Check sheet for the drawn part. Datum: minimum x, y, z corner. Units: mm. A direction names the side the tool comes from. Give positions to 0.01 mm unless a question says otherwise; leave off trailing zeros. Order: outer loops, then holes, each group sorted by start corner. A loop starts at its lowest first (then second) coordinate and runs counter-clockwise, first axis right, second up.
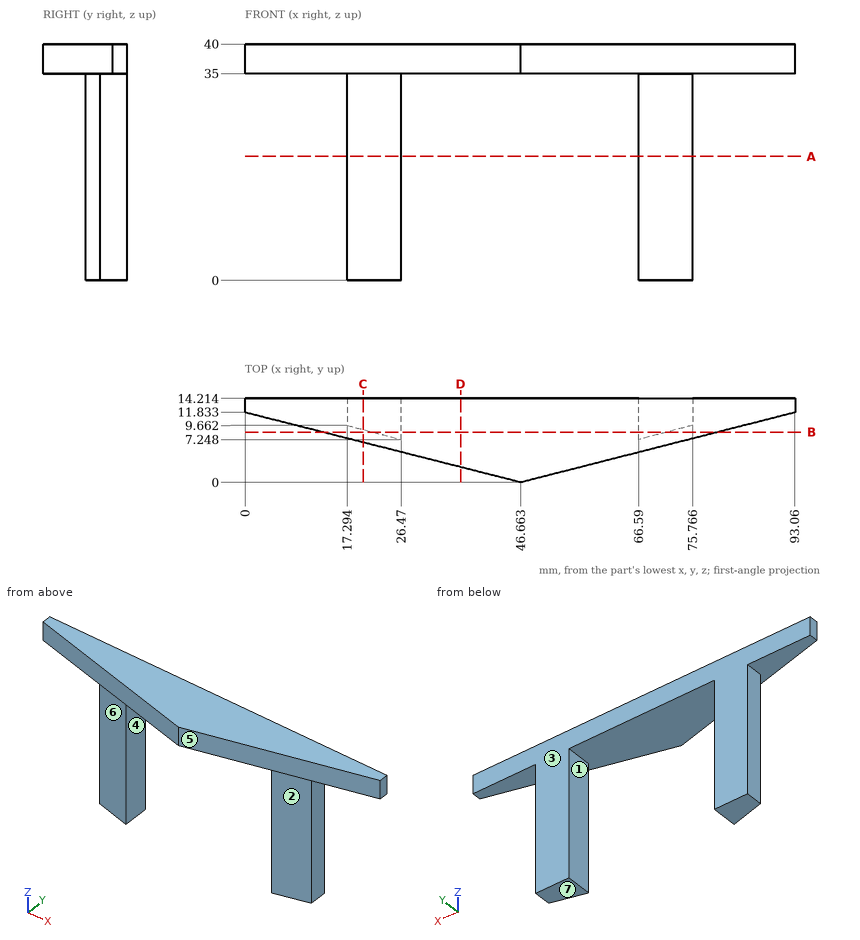
(1) Section check D-D, the plane x = 36.5. Enter the section's corners in (y, z), then the cut area to 3 significant figures.
Solved:
outline: (2.58, 35) - (14.21, 35) - (14.21, 40) - (2.58, 40) - close
area: 58.2 mm2
(2) Section check C-C, the plane x = 20. Enter the section's corners in (y, z).
Solved:
outline: (6.76, 35) - (8.95, 35) - (8.95, 0) - (14.21, 0) - (14.21, 40) - (6.76, 40) - close
(3) Set-up check for the marked faces 1, 2 and 3: record each of +Z, -Z, +X, -X, +Y, -Y from which the full face is reachable in a straight line by a thin tool's end or side.
Solved:
face 1: -Z, +Y, -Y
face 2: -Z, +X, -Y
face 3: +Z, -Z, +X, -X, +Y
(4) Section check A-A, the plane z = 21. Enter the section's corners in (x, y) (1 decimal), then the cut area to 3 significant figures.
Solved:
outline: (17.3, 9.7) - (26.5, 7.2) - (26.5, 14.2) - (17.3, 14.2) - close; (66.6, 7.2) - (75.8, 9.7) - (75.8, 14.2) - (66.6, 14.2) - close
area: 106 mm2
(5) Scan lines: line 1 (X direction, y = 12.5, z = 25.5) (1 decimal); line 2 (Z direction, x = 61, y = 5); line 3 (Y direction, x = 25.5, z = 30). Record each from-to range of solid material in increasing order.
Solved:
line 1: x = 17.3 to 26.5, 66.6 to 75.8
line 2: z = 35 to 40
line 3: y = 7.5 to 14.21
(6) Release check for a two-part mould opening along X. For the marked faces 4, 5, 6 and 7 record: pulls with the +X half, pulls with the -X half, needs draft (parallel to the pull), parting line crosses it, or undercut.
Solved:
face 4: undercut
face 5: pulls with the +X half
face 6: pulls with the -X half
face 7: needs draft
(7) Go/stop test with flat-tipped pins: pin 1 (3.5 mm diameter, centred on y = 12.5, z = 13.5, fed in from -X); pin 2 (5.5 mm diameter, centred on y = 11, z = 10.5, fed in from +X); pin 3 (4.5 mm diameter, centred on x = 54, y = 5, fed in from -Z). Record where each tip stops, or that it passes through.
Solved:
pin 1: stops at x = 17.29
pin 2: stops at x = 75.77
pin 3: stops at z = 35
(8) Section check B-B, the plane y = 8.5. Enter the section's corners in (x, z) (1 decimal).
Solved:
outline: (13.1, 35) - (21.7, 35) - (21.7, 0) - (26.5, 0) - (26.5, 35) - (66.6, 35) - (66.6, 0) - (71.3, 0) - (71.3, 35) - (80, 35) - (80, 40) - (13.1, 40) - close
